Could you check a few things on this model? Use its own coordinates, in mm. Round coordinates to 2 decimals unless told otherwise and drop trailing zeros. Loops run counter-clockwise (first coordinate to the right, second up) from the corner with the lowest first, then second, coordinate; pieces in that order, holes last.
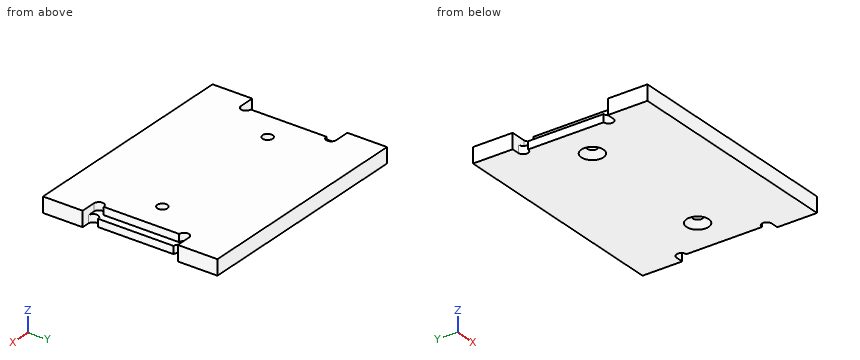
Solid Edge part; units mm, degrees
sketch "Sketch1" plane through (0, 0, 0) normal (0, 0, 1) x (1, 0, 0)
  line L0 (-36.25, 27.5) -> (36.25, 27.5)
  line L1 (36.25, 27.5) -> (36.25, -27.5)
  line L2 (36.25, -27.5) -> (-36.25, -27.5)
  line L3 (-36.25, -27.5) -> (-36.25, 27.5)
extrude "ExtrudedProtrusion_7" add sketch "Sketch1" along normal blind 4.8
sketch "Sketch2" plane through (0, 0, 4.8) normal (0, 0, 1) x (1, 0, 0)
  line L0 (-33.85, -15) -> (-31.45, -15)
  line L1 (-31.45, -11.9) -> (-31.45, 11.9)
  line L2 (-33.85, 15) -> (-31.45, 15)
  line L3 (-33.85, 15) -> (-33.85, -15)
  arc A0 (-31.45, -11.9) -> (-31.45, -15) centre (-31.45, -13.45) cw
  arc A1 (-31.45, 15) -> (-31.45, 11.9) centre (-31.45, 13.45) cw
  line L4 (31.45, -15) -> (33.85, -15)
  line L5 (33.85, -15) -> (33.85, 15)
  line L6 (33.85, 15) -> (31.45, 15)
  line L7 (31.45, 11.9) -> (31.45, -11.9)
  arc A2 (31.45, 11.9) -> (31.45, 15) centre (31.45, 13.45) cw
  arc A3 (31.45, -15) -> (31.45, -11.9) centre (31.45, -13.45) cw
extrude "ExtrudedCutout_13" cut sketch "Sketch2" against normal blind 2.4
sketch "Sketch3" plane through (0, 0, 4.8) normal (0, 0, 1) x (1, 0, 0)
  line L0 (-33.85, 11.9) -> (-33.85, -11.9)
  line L1 (-36.25, -15) -> (-33.85, -15)
  line L2 (-36.25, 15) -> (-36.25, -15)
  line L3 (-36.25, 15) -> (-33.85, 15)
  arc A0 (-33.85, 15) -> (-33.85, 11.9) centre (-33.85, 13.45) cw
  arc A1 (-33.85, -11.9) -> (-33.85, -15) centre (-33.85, -13.45) cw
  line L4 (36.25, 15) -> (33.85, 15)
  line L5 (36.25, -15) -> (36.25, 15)
  line L6 (33.85, -15) -> (36.25, -15)
  line L7 (33.85, 11.9) -> (33.85, -11.9)
  arc A2 (33.85, 11.9) -> (33.85, 15) centre (33.85, 13.45) cw
  arc A3 (33.85, -15) -> (33.85, -11.9) centre (33.85, -13.45) cw
extrude "ExtrudedCutout_14" cut sketch "Sketch3" against normal blind 4.8
hole "Hole_5" at (-22.5, 0, 0) direction (0, 0, 1) diameter 3.2 end up to next countersink diameter 6.94 countersink angle 90
hole "Hole1" at (22.5, 0, 0) direction (0, 0, 1) diameter 3.2 end up to next countersink diameter 6.94 countersink angle 90
properties material "Polycarbonate"
Item 1: If we section it at D-D, the plane y = -13.45: Please give me the cut outline in (x, z), then the cut area to 3 significant figures.
Results list:
outline: (-32.3, 0) - (32.3, 0) - (32.3, 2.4) - (29.9, 2.4) - (29.9, 4.8) - (-29.9, 4.8) - (-29.9, 2.4) - (-32.3, 2.4) - close
area: 299 mm2
Item 2: If we section it at B-B, the plane z = 1: Please give me the cut outline in (x, y), then the cut area to 3 significant figures.
Results list:
outline: (-36.25, -27.5) - (36.25, -27.5) - (36.25, -15) - (33.85, -15) arc R1.55 cw to (33.85, -11.9) - (33.85, 11.9) arc R1.55 cw to (33.85, 15) - (36.25, 15) - (36.25, 27.5) - (-36.25, 27.5) - (-36.25, 15) - (-33.85, 15) arc R1.55 cw to (-33.85, 11.9) - (-33.85, -11.9) arc R1.55 cw to (-33.85, -15) - (-36.25, -15) - close; hole circle Ø4.94 at (-22.5, 0); hole circle Ø4.94 at (22.5, 0)
area: 3,790 mm2
Item 3: If we section it at C-C, the plane y = 0: Please give me the cut outline in (x, z), then the cut area to 3 significant figures.
Results list:
outline: (-33.85, 0) - (-25.97, 0) - (-24.1, 1.87) - (-24.1, 4.8) - (-31.45, 4.8) - (-31.45, 2.4) - (-33.85, 2.4) - close; (-20.9, 1.87) - (-19.03, 0) - (19.03, 0) - (20.9, 1.87) - (20.9, 4.8) - (-20.9, 4.8) - close; (24.1, 1.87) - (25.97, 0) - (33.85, 0) - (33.85, 2.4) - (31.45, 2.4) - (31.45, 4.8) - (24.1, 4.8) - close
area: 276 mm2
Item 4: If we section it at A-A, the plane x = 22.5: Please give me the cut outline in (y, z), then the cut area to 3 significant figures.
Results list:
outline: (-27.5, 0) - (-3.47, 0) - (-1.6, 1.87) - (-1.6, 4.8) - (-27.5, 4.8) - close; (1.6, 1.87) - (3.47, 0) - (27.5, 0) - (27.5, 4.8) - (1.6, 4.8) - close
area: 245 mm2
Item 5: If I drill on line 1 along X through (y, z) = (0, 2.5); line 2 along Y through (x, z) = (22.5, 3.75); line 3 along Z through (x, y) = (31.5, 10.5), over which ranges is the centre line in solid material (lowest first)?
Results list:
line 1: x = -31.45 to -24.1, -20.9 to 20.9, 24.1 to 31.45
line 2: y = -27.5 to -1.6, 1.6 to 27.5
line 3: z = 0 to 2.4
Item 6: Will these pins go through, and if not, where does the flat tip stop? pin 1 (1.9 mm diameter, centred on x = 22.5, y = 0, fed in from -Z); pin 2 (2.5 mm diameter, centred on y = -1, z = 1.5, fed in from -X); pin 3 (0.7 mm diameter, centred on y = -1.5, z = 3.5, fed in from +X); pin 4 (2 mm diameter, centred on y = 11.5, z = 3.5, fed in from -X).
Results list:
pin 1: passes through
pin 2: stops at x = -33.85
pin 3: stops at x = 31.45
pin 4: stops at x = -31.45
